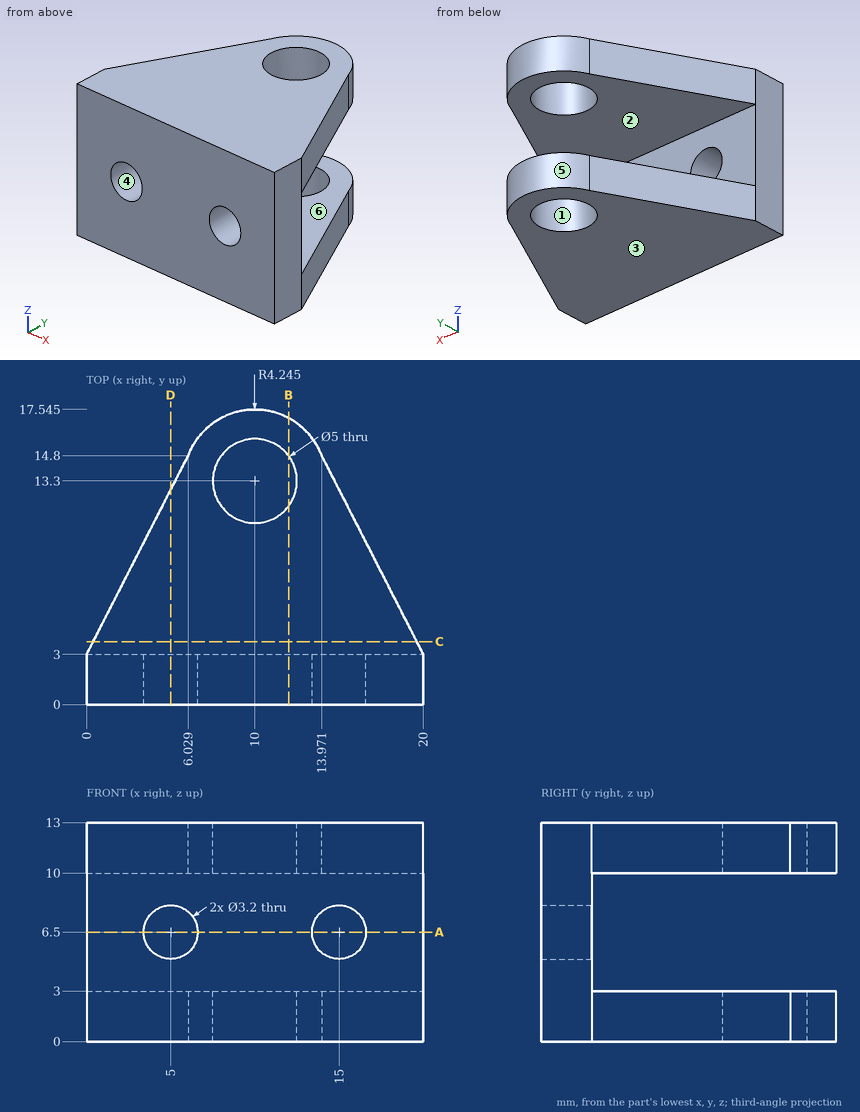
Geometry: see drawing. Coordinates: mm, zero at the bounding-box minimum. A direction names the side the tool comes from. Coordinates: 2 decimals unless noted, no trailing zeros. Loops run counter-clockwise (first coordinate to the right, second up) from the corner with the lowest first, then second, coordinate; pieces in that order, holes last. Notation, with made-up numbers: M -5,46 L 49,46 A7 ccw 49,54 Z; hole C 78,27 d2. An arc over 180 degrees is marked long. Answer in a Markdown table with one row per item.
Q1. Draft query along Z for the marked faces 1, 2, 3 and 4. Return one class per face: pulls with the +Z half, pulls with the -Z half, needs draft (parallel to the pull), parting line crosses it, or undercut.
Answers below:
| item | result |
|---|---|
| face 1 | needs draft |
| face 2 | undercut |
| face 3 | pulls with the -Z half |
| face 4 | undercut |
Q2. Section A-A on z = 6.5. Return the cut outline in (x, y).
Answers below:
| item | result |
|---|---|
| outline | M 0,0 L 3.4,0 L 3.4,3 L 0,3 Z; M 6.6,0 L 13.4,0 L 13.4,3 L 6.6,3 Z; M 16.6,0 L 20,0 L 20,3 L 16.6,3 Z |
Q3. Ray query, probe 1 along X at (y, z) = (1.8, 6.5); probe 2 along Z at (x, y) = (10, 16); probe 3 along Z at (x, y) = (5, 1.05). Return the intervals inside material, ascending. Write a range as from..to.
Answers below:
| item | result |
|---|---|
| probe 1 | x = 0..3.4, 6.6..13.4, 16.6..20 |
| probe 2 | z = 0..3, 10..13 |
| probe 3 | z = 0..4.9, 8.1..13 |
Q4. Set-up query: the marked faces 5 and 6. Return all of +Z, -Z, +X, -X, +Y, -Y with unobstructed straight access to the full face (end or side cutting, diameter ignored); none if empty.
Answers below:
| item | result |
|---|---|
| face 5 | +Z, -Z, +Y |
| face 6 | +X, -X, +Y |
Q5. Section C-C on y = 3.75. Return the cut outline in (x, z).
Answers below:
| item | result |
|---|---|
| outline | M 0.38,0 L 19.62,0 L 19.62,3 L 0.38,3 Z; M 0.38,10 L 19.62,10 L 19.62,13 L 0.38,13 Z |
Q6. First-contact query: pin 1 (4 mm diameter, centred on x = 15, z = 6.5, fed in from +Y); pin 2 (3 mm diameter, centred on x = 10, y = 13.3, fed in from -Z); pin 3 (3 mm diameter, centred on x = 3.5, z = 1.5, fed in from -Y). Flat tips, straight axial feed; report the tip coordinate or a pass-through.
Answers below:
| item | result |
|---|---|
| pin 1 | stops at y = 3 |
| pin 2 | passes through |
| pin 3 | stops at y = 0 |
Q7. Section D-D on x = 5. Return the cut outline in (y, z).
Answers below:
| item | result |
|---|---|
| outline | M 0,0 L 12.79,0 L 12.79,3 L 3,3 L 3,4.9 L 0,4.9 Z; M 0,8.1 L 3,8.1 L 3,10 L 12.79,10 L 12.79,13 L 0,13 Z |
Q8. Section B-B on x = 12. Return the cut outline in (y, z).
Answers below:
| item | result |
|---|---|
| outline | M 0,0 L 11.8,0 L 11.8,3 L 3,3 L 3,10 L 11.8,10 L 11.8,13 L 0,13 Z; M 14.8,0 L 17.04,0 L 17.04,3 L 14.8,3 Z; M 14.8,10 L 17.04,10 L 17.04,13 L 14.8,13 Z |
